Check sheet for the modelled part. Datum: model origin and axes. Units: mm. Face numbers are marked on the shaded views. A direction names the side the tool comes from. Round coordinates to 2 decimals unless told otherwise and drop trailing zeros. Order: outer loops, then holes, each group sorted by start corner. A loop starts at its lowest first (then second) coordinate and runs counter-clockwise, first axis right, second up. Notation, with made-up numbers: (80, 23) -> (85, 23) arc R26 ccw to (85, 61) -> close; hole circle Ø3 at (71.25, 63). An arc over 180 degrees is marked (long way). Answer in a Markdown table with one row per item.
from build123d import *

# Parameters (mm, degrees)
CUBE005_W                     = 5.1
CUBE005_H                     = 5.2
CUBE005_DEPTH                 = 2
CYLINDER003_R                 = 1.3
CYLINDER003_DEPTH             = 7.1
CUBE001_W                     = 4.4
CUBE001_H                     = 5
CUBE001_DEPTH                 = 7
CYLINDER002_R                 = 2.2
CYLINDER002_DEPTH             = 7
DIFFERENCE001_PLACEMENT_ANGLE = 90
CYLINDER005_R                 = 1.3
CYLINDER005_DEPTH             = 7.1
CUBE002_W                     = 4.4
CUBE002_H                     = 5
CUBE002_DEPTH                 = 7
CYLINDER004_R                 = 2.2
CYLINDER004_DEPTH             = 7
DIFFERENCE002_PLACEMENT_ANGLE = 90
CYLINDER007_R                 = 1.3
CYLINDER007_DEPTH             = 7.1
CUBE003_W                     = 4.4
CUBE003_H                     = 5
CUBE003_DEPTH                 = 7
CYLINDER006_R                 = 2.2
CYLINDER006_DEPTH             = 7
DIFFERENCE003_PLACEMENT_ANGLE = 90
CUBE004_W                     = 24.75
CUBE004_H                     = 21.5
CUBE004_DEPTH                 = 7
CYLINDER001_R                 = 1.3
CYLINDER001_DEPTH             = 7.1
CUBE_W                        = 4.4
CUBE_H                        = 5
CUBE_DEPTH                    = 7
CYLINDER_R                    = 2.2
CYLINDER_DEPTH                = 7
DIFFERENCE_PLACEMENT_ANGLE    = 90
FILLET_R                      = 1


with BuildPart() as cube005:
    # cube005 → cube005 (new body)
    with BuildSketch(Plane(origin=(8.8, 1.35, -0.01), x_dir=(1, 0, 0), z_dir=(0, 0, 1))):
        with Locations((2.55, 2.6)):
            Rectangle(CUBE005_W, CUBE005_H)
    extrude(amount=CUBE005_DEPTH)


with BuildPart() as cylinder003:
    # cylinder003 → cylinder003 (new body)
    with BuildSketch(Plane.XY.offset(-0.01)):
        Circle(CYLINDER003_R)
    extrude(amount=CYLINDER003_DEPTH)


with BuildPart() as cube001:
    # cube001 → cube001 (new body)
    with BuildSketch(Plane(origin=(-2.2, 0, 0), x_dir=(1, 0, 0), z_dir=(0, 0, 1))):
        with Locations((2.2, 2.5)):
            Rectangle(CUBE001_W, CUBE001_H)
    extrude(amount=CUBE001_DEPTH)


with BuildPart() as difference001:
    # cylinder002 → cylinder002 (new body)
    with BuildSketch(Plane.XY):
        Circle(CYLINDER002_R)
    extrude(amount=CYLINDER002_DEPTH)

    # union001: union cube001
    add(cube001.part)

    # difference001: cut cylinder003
    add(cylinder003.part, mode=Mode.SUBTRACT)


with BuildPart() as difference001_1:
    # difference001 placement: moved
    add(difference001.part.moved(Location((29.6, 0, 0))).rotate(Axis((29.6, 0, 0), (0, 0, 1)), DIFFERENCE001_PLACEMENT_ANGLE))


with BuildPart() as cylinder005:
    # cylinder005 → cylinder005 (new body)
    with BuildSketch(Plane.XY.offset(-0.01)):
        Circle(CYLINDER005_R)
    extrude(amount=CYLINDER005_DEPTH)


with BuildPart() as cube002:
    # cube002 → cube002 (new body)
    with BuildSketch(Plane(origin=(-2.2, 0, 0), x_dir=(1, 0, 0), z_dir=(0, 0, 1))):
        with Locations((2.2, 2.5)):
            Rectangle(CUBE002_W, CUBE002_H)
    extrude(amount=CUBE002_DEPTH)


with BuildPart() as difference002:
    # cylinder004 → cylinder004 (new body)
    with BuildSketch(Plane.XY):
        Circle(CYLINDER004_R)
    extrude(amount=CYLINDER004_DEPTH)

    # union002: union cube002
    add(cube002.part)

    # difference002: cut cylinder005
    add(cylinder005.part, mode=Mode.SUBTRACT)


with BuildPart() as difference002_1:
    # difference002 placement: moved
    add(difference002.part.moved(Location((29.6, 17.1, 0))).rotate(Axis((29.6, 17.1, 0), (0, 0, 1)), DIFFERENCE002_PLACEMENT_ANGLE))


with BuildPart() as cylinder007:
    # cylinder007 → cylinder007 (new body)
    with BuildSketch(Plane.XY.offset(-0.01)):
        Circle(CYLINDER007_R)
    extrude(amount=CYLINDER007_DEPTH)


with BuildPart() as cube003:
    # cube003 → cube003 (new body)
    with BuildSketch(Plane(origin=(-2.2, 0, 0), x_dir=(1, 0, 0), z_dir=(0, 0, 1))):
        with Locations((2.2, 2.5)):
            Rectangle(CUBE003_W, CUBE003_H)
    extrude(amount=CUBE003_DEPTH)


with BuildPart() as difference003:
    # cylinder006 → cylinder006 (new body)
    with BuildSketch(Plane.XY):
        Circle(CYLINDER006_R)
    extrude(amount=CYLINDER006_DEPTH)

    # union003: union cube003
    add(cube003.part)

    # difference003: cut cylinder007
    add(cylinder007.part, mode=Mode.SUBTRACT)


with BuildPart() as difference003_1:
    # difference003 placement: moved
    add(difference003.part.moved(Location((0, 17.1, 0))).rotate(Axis((0, 17.1, 0), (0, 0, -1)), DIFFERENCE003_PLACEMENT_ANGLE))


with BuildPart() as cube004:
    # cube004 → cube004 (new body)
    with BuildSketch(Plane(origin=(2.5, -2.2, 0), x_dir=(1, 0, 0), z_dir=(0, 0, 1))):
        with Locations((12.375, 10.75)):
            Rectangle(CUBE004_W, CUBE004_H)
    extrude(amount=CUBE004_DEPTH)


with BuildPart() as cylinder001:
    # cylinder001 → cylinder001 (new body)
    with BuildSketch(Plane.XY.offset(-0.01)):
        Circle(CYLINDER001_R)
    extrude(amount=CYLINDER001_DEPTH)


with BuildPart() as cube:
    # cube → cube (new body)
    with BuildSketch(Plane(origin=(-2.2, 0, 0), x_dir=(1, 0, 0), z_dir=(0, 0, 1))):
        with Locations((2.2, 2.5)):
            Rectangle(CUBE_W, CUBE_H)
    extrude(amount=CUBE_DEPTH)


with BuildPart() as fillet_body:
    # cylinder → cylinder (new body)
    with BuildSketch(Plane.XY):
        Circle(CYLINDER_R)
    extrude(amount=CYLINDER_DEPTH)

    # union: union cube
    add(cube.part)

    # difference: cut cylinder001
    add(cylinder001.part, mode=Mode.SUBTRACT)


with BuildPart() as fillet_body_1:
    # difference placement: moved
    add(fillet_body.part.rotate(Axis((0, 0, 0), (0, 0, -1)), DIFFERENCE_PLACEMENT_ANGLE))

    # union004: union difference001, difference002, difference003, cube004
    add(difference001_1.part)
    add(difference002_1.part)
    add(difference003_1.part)
    add(cube004.part)

    # difference004: cut cube005
    add(cube005.part, mode=Mode.SUBTRACT)

    # Fillet
    fillet_edges = [fillet_body_1.edges().sort_by_distance(p)[0] for p in [
        (2.5, 2.2, 3.5),
        (2.5, 14.9, 3.5),
        (27.25, 14.9, 3.5),
        (27.25, 2.2, 3.5),
        (13.9, 1.35, 0.995),
        (11.35, 1.35, 1.99),
        (8.8, 1.35, 0.995),
        (13.9, 3.95, 1.99),
        (13.9, 6.55, 0.995),
        (11.35, 6.55, 1.99),
        (8.8, 6.55, 0.995),
        (8.8, 3.95, 1.99),
    ]]
    fillet(fillet_edges, radius=FILLET_R)


solid = fillet_body_1.part
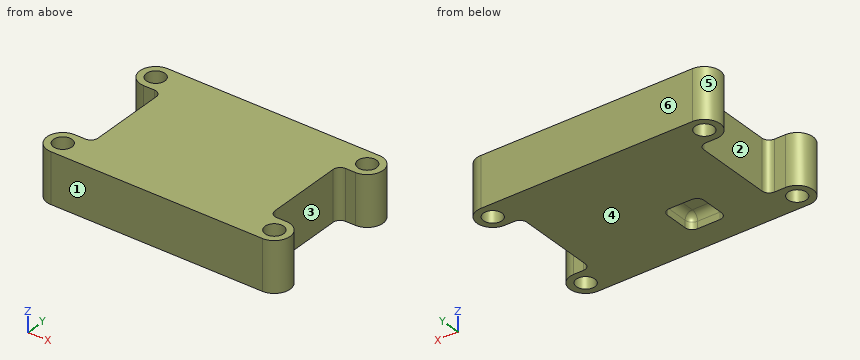
Item 1: Cross-section at C-C (y = -0.5). Record the boundary of the cut face in (x, z), and give its area (3 significant figures).
Result sheet:
| item | result |
|---|---|
| outline | (-2.14, 0) -> (-1.2, 0) -> (-1.2, 7) -> (-2.14, 7) -> close; (1.2, 0) -> (28.4, 0) -> (28.4, 7) -> (1.2, 7) -> close; (30.8, 0) -> (31.74, 0) -> (31.74, 7) -> (30.8, 7) -> close |
| area | 204 mm^2 |
Item 2: Depth check by flat-ended pin: P1, Ø0.5, axis at y = 3.5, z = 0.5, coming from the +X side; P2, Ø2, axis at y = 8, z = 2, coming from the -X side; P3, Ø2, axis at x = 0, y = 0, coming from the +Z side; P4, Ø1.6, axis at x = 11.5, y = 3, coming from the -Z side. Enter the tip coordinate at first touch or a pass-through.
Result sheet:
| item | result |
|---|---|
| P1 | stops at x = 27.25 |
| P2 | stops at x = 2.5 |
| P3 | passes through |
| P4 | stops at z = 1.98 |
Item 3: Cross-section at B-B (z = 0.5). Record the boundary of the cut face in (x, y), and give its area (3 significant figures).
Result sheet:
| item | result |
|---|---|
| outline | (0, -2.2) -> (29.6, -2.2) arc R2.2 ccw to (29.6, 2.2) -> (28.25, 2.2) arc R1 cw to (27.25, 3.2) -> (27.25, 13.9) arc R1 cw to (28.25, 14.9) -> (29.6, 14.9) arc R2.2 ccw to (29.6, 19.3) -> (0, 19.3) arc R2.2 ccw to (0, 14.9) -> (1.5, 14.9) arc R1 cw to (2.5, 13.9) -> (2.5, 3.2) arc R1 cw to (1.5, 2.2) -> (0, 2.2) arc R2.2 ccw to start; hole circle Ø2.6 at (0, 0); hole circle Ø2.6 at (0, 17.1); hole (8.8, 2.35) arc R1 ccw to (9.8, 1.35) -> (12.9, 1.35) arc R1 ccw to (13.9, 2.35) -> (13.9, 5.55) arc R1 ccw to (12.9, 6.55) -> (9.8, 6.55) arc R1 ccw to (8.8, 5.55) -> close; hole circle Ø2.6 at (29.6, 0); hole circle Ø2.6 at (29.6, 17.1) |
| area | 559 mm^2 |
Item 4: Cross-section at A-A (x = 0.5). Record the boundary of the cut face in (y, z), and give its area (3 significant figures).
Result sheet:
| item | result |
|---|---|
| outline | (-2.2, 0) -> (-1.2, 0) -> (-1.2, 7) -> (-2.2, 7) -> close; (1.2, 0) -> (2.2, 0) -> (2.2, 7) -> (1.2, 7) -> close; (14.9, 0) -> (15.9, 0) -> (15.9, 7) -> (14.9, 7) -> close; (18.3, 0) -> (19.3, 0) -> (19.3, 7) -> (18.3, 7) -> close |
| area | 28.0 mm^2 |
Item 5: Scan lines: line 1 (X direction, y = 17.1, z = 4); line 2 (Y direction, x = 28.5, z = 0.75); line 3 (X direction, y = 16, z = 5). Record each from-to range of solid material in increasing order. Write a range as [from, to].
Result sheet:
| item | result |
|---|---|
| line 1 | x = [-2.2, -1.3], [1.3, 28.3], [30.9, 31.8] |
| line 2 | y = [-2.2, -0.69], [0.69, 2.2], [14.9, 16.41], [17.79, 19.3] |
| line 3 | x = [-1.91, -0.69], [0.69, 28.91], [30.29, 31.51] |
Item 6: Mould release check, pull along Y, two halves, no side actions. Record for the marked faces 4, 5 and 6: pulls with the +Y half, pulls with the -Y half, needs draft (parallel to the pull), parting line crosses it, or undercut.
Result sheet:
| item | result |
|---|---|
| face 4 | needs draft |
| face 5 | undercut |
| face 6 | pulls with the +Y half |
Item 7: Cross-section at D-D (z = 4.5). Record the boundary of the cut face in (x, y), and give its area (3 significant figures).
Result sheet:
| item | result |
|---|---|
| outline | (0, -2.2) -> (29.6, -2.2) arc R2.2 ccw to (29.6, 2.2) -> (28.25, 2.2) arc R1 cw to (27.25, 3.2) -> (27.25, 13.9) arc R1 cw to (28.25, 14.9) -> (29.6, 14.9) arc R2.2 ccw to (29.6, 19.3) -> (0, 19.3) arc R2.2 ccw to (0, 14.9) -> (1.5, 14.9) arc R1 cw to (2.5, 13.9) -> (2.5, 3.2) arc R1 cw to (1.5, 2.2) -> (0, 2.2) arc R2.2 ccw to start; hole circle Ø2.6 at (0, 0); hole circle Ø2.6 at (0, 17.1); hole circle Ø2.6 at (29.6, 0); hole circle Ø2.6 at (29.6, 17.1) |
| area | 585 mm^2 |
Item 8: Set-up check for the marked faces 1, 2 and 3: record each of +Z, -Z, +X, -X, +Y, -Y from which the full face is reachable in a straight line by a thin tool's end or side.
Result sheet:
| item | result |
|---|---|
| face 1 | +Z, -Z, +X, -X, -Y |
| face 2 | +Z, -Z, -X |
| face 3 | +Z, -Z, +X |
